Check sheet for the modelled part. Datum: model origin and axes. Units: mm. A direction names the side the tool comes from. Round coordinates to 2 decimals unless told otherwise and drop trailing zeros. Order: outer loops, then holes, each group sorted by start corner. A loop starts at its lowest first (then second) coordinate and runs counter-clockwise, first axis right, second up.
```python
from build123d import *

# Parameters (mm, degrees)
ESBO_O1_R                = 3.15
ESBO_O1_R_2              = 1.6
RESSALTO_EXTRUS_O1_DEPTH = 6
FILETE3_R                = 4
ESBO_O2_W                = 20.15
ESBO_O2_H                = 7.319150415
CORTE_EXTRUS_O1_DEPTH    = 10
FILETE2_R                = 8


with BuildPart() as part:
    # Esboço1 → Ressalto-extrusão1 (new body)
    with BuildSketch(Plane.XY):
        Polygon((20.5, 0), (9, 0), (9, -19), (0, -19), (0, -29), (6, -29), (6, -39), (0, -39), (0, -45), (29.15, -45), (29.15, -15), (42, -15), (42, 0), (30.5, 0), (30.5, 6), (20.5, 6), align=None)
        with Locations((19.15, -27.680849585)):
            Circle(ESBO_O1_R, mode=Mode.SUBTRACT)
        with Locations((16, -8)):
            Circle(ESBO_O1_R_2, mode=Mode.SUBTRACT)
        with Locations((36, -8)):
            Circle(ESBO_O1_R_2, mode=Mode.SUBTRACT)
    extrude(amount=RESSALTO_EXTRUS_O1_DEPTH)

    # Filete3
    filete3_edges = [part.edges().sort_by_distance(p)[0] for p in [
        (29.15, -15, 3),
    ]]
    fillet(filete3_edges, radius=FILETE3_R)

    # Esboço2 → Corte-extrusão1 (cut)
    with BuildSketch(Plane.XY.offset(6)):
        Polygon((9, -19), (0, -19), (0, -29), (6, -29), (6, -39), (0, -39), (0, -45), (9, -45), (9, -37.680849585), align=None)
        with Locations((19.075, -41.340424793)):
            Rectangle(ESBO_O2_W, ESBO_O2_H)
    extrude(amount=-CORTE_EXTRUS_O1_DEPTH, mode=Mode.SUBTRACT)

    # Filete2
    filete2_edges = [part.edges().sort_by_distance(p)[0] for p in [
        (42, -15, 3),
        (9, -37.680849585, 3),
        (29.15, -37.680849585, 3),
    ]]
    fillet(filete2_edges, radius=FILETE2_R)


solid = part.part
```
Item 1: Release check for a two-part mould opening along Y. For faces 1 (the flat face through (33.6, -15, 3)), 2 (the flat face through (29.15, -24, 3)), 3 (the cylindrical face through (34.4, -7.93, 2.96)), 4 (the flat face through (15, 0, 3)) record: released by +Y, released by -Y, zero draft, split by the parting line, or undercut.
Answer:
face 1: released by -Y
face 2: zero draft
face 3: undercut
face 4: released by +Y
Item 2: Sectioned sample at B-B (y = -25). Record the cut outline in (x, z).
Answer:
outline: (9, 0) - (17.5, 0) - (17.5, 6) - (9, 6) - close; (20.8, 0) - (29.15, 0) - (29.15, 6) - (20.8, 6) - close
Item 3: Sectioned sample at D-D (y = -8). Record the cut outline in (x, z).
Answer:
outline: (9, 0) - (14.4, 0) - (14.4, 6) - (9, 6) - close; (17.6, 0) - (34.4, 0) - (34.4, 6) - (17.6, 6) - close; (37.6, 0) - (41.94, 0) - (41.94, 6) - (37.6, 6) - close
Item 4: Sectioned sample at C-C (z = 4.4). Record the cut outline in (x, y).
Answer:
outline: (9, -29.68) arc R8 ccw to (17, -37.68) - (21.15, -37.68) arc R8 ccw to (29.15, -29.68) - (29.15, -19) arc R4 cw to (33.15, -15) - (34, -15) arc R8 ccw to (42, -7) - (42, 0) - (30.5, 0) - (30.5, 6) - (20.5, 6) - (20.5, 0) - (9, 0) - close; hole circle Ø3.2 at (16, -8); hole circle Ø6.3 at (19.15, -27.68); hole circle Ø3.2 at (36, -8)
Item 5: Access from +Z, -Z, +X, -X, +Y, -Y to the whole of each face (thin tool, end or side, straight path). Record for faces 5 (the flat face through (30.5, 3, 3)), 6 (the flat face through (9, -15, 3)), 7 (the flat face through (20.5, 3, 3)).
Answer:
face 5: +Z, -Z, +X, +Y
face 6: +Z, -Z, -X, +Y, -Y
face 7: +Z, -Z, -X, +Y
Item 6: Go/stop test with flat-tipped pins: P1, Ø1.8, axis at x = 15, z = 1.5, coming from the +Y side; P2, Ø1.9, axis at x = 36, y = -8, coming from the +Z side; P3, Ø1.8, axis at y = 3.5, z = 4, coming from the +X side. Record where each tip stops, or that it passes through.
Answer:
P1: stops at y = 0
P2: passes through
P3: stops at x = 30.5
Item 7: Sectioned sample at A-A (x = 19.15). Record the cut outline in (y, z), and give its area (3 significant figures).
Answer:
outline: (-37.68, 0) - (-30.83, 0) - (-30.83, 6) - (-37.68, 6) - close; (-24.53, 0) - (0, 0) - (0, 6) - (-24.53, 6) - close
area: 188 mm2
Item 8: Scan lines: line 1 along Y through (x, z) = (19.15, 3.85); line 2 along X through (y, z) = (-20.5, 1.1); line 3 along X through (y, z) = (-9, 4.55). Record each from-to range of solid material in increasing order.
Answer:
line 1: y = -37.68 to -30.83, -24.53 to 0
line 2: x = 9 to 29.15
line 3: x = 9 to 14.75, 17.25 to 34.75, 37.25 to 41.75
